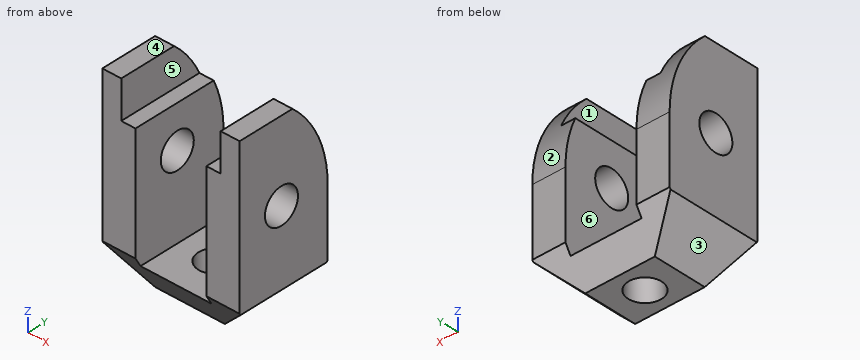
```python
from build123d import *

# Parameters (mm, degrees)
SKETCH1_R                           = 7.5
BOSS_EXTRUDE1_DEPTH                 = 58
CUT_EXTRUDE1_DEPTH                  = 107.60206377
CUT_EXTRUDE1_DEPTH_BACK             = 10
SKETCH3_W                           = 30
SKETCH3_H                           = 53
CUT_EXTRUDE3_DEPTH                  = 107.60206377
CUT_EXTRUDE3_DIRECTION_2_REACH      = 108.602
CUT_EXTRUDE3_DIRECTION_2_END_RADIUS = 50
CUT_EXTRUDE4_DEPTH                  = 107.60206377
SKETCH8_R                           = 7
CUT_EXTRUDE5_DEPTH                  = 107.60206377


with BuildPart() as part:
    # Sketch1 → Boss-Extrude1 (new body)
    with BuildSketch(Plane(origin=(0, 0, 0), x_dir=(0, 0, -1), z_dir=(1, 0, 0))):
        with BuildLine():
            Line((0, 0), (65, 0))
            Line((65, 0), (80, 8.660254038))
            Line((80, 8.660254038), (80, 31.339745962))
            Line((80, 31.339745962), (65, 40))
            Line((65, 40), (36.66060556, 40))
            ThreePointArc((36.66060556, 40), (16.66060556, 35.82575695), (0, 24))
            Line((0, 24), (0, 0))
        make_face()
        with Locations(Location((34, 19, 0), (0, 0, 180))):
            Circle(SKETCH1_R, mode=Mode.SUBTRACT)
    extrude(amount=BOSS_EXTRUDE1_DEPTH)

    # Sketch3 → Cut-Extrude1 (cut, two sides: drawn at the far end of the back side and taken through both)
    with BuildSketch(Plane(origin=(0, 0, 0), x_dir=(1, 0, 0), z_dir=(0, 1, 0)).offset(-CUT_EXTRUDE1_DEPTH_BACK)):
        with Locations((29, 42.5)):
            Rectangle(SKETCH3_W, SKETCH3_H)
    extrude(amount=CUT_EXTRUDE1_DEPTH + CUT_EXTRUDE1_DEPTH_BACK, mode=Mode.SUBTRACT)

    # Sketch5 → Cut-Extrude3 (cut)
    with BuildSketch(Plane(origin=(0, 0, 0), x_dir=(1, 0, 0), z_dir=(0, 1, 0))):
        Polygon((29, 0), (29, 16), (14, 16), (8, 16), (8, 0), align=None)
        Polygon((44, 16), (29, 16), (29, 0), (50, 0), (50, 16), align=None)
    extrude(amount=-CUT_EXTRUDE3_DEPTH, mode=Mode.SUBTRACT)

    # Cut-Extrude3 direction 2: up to this cylinder (the profile starts inside it)
    cut_extrude3_direction_2_end = Plane(origin=(29, -10, -36.66060556), z_dir=(-1, 0, 0)) * Cylinder(CUT_EXTRUDE3_DIRECTION_2_END_RADIUS, 339.204, mode=Mode.PRIVATE)
    # Sketch5 → Cut-Extrude3 direction 2 (cut, up to the surface)
    with BuildSketch(Plane(origin=(0, 0, 0), x_dir=(1, 0, 0), z_dir=(0, 1, 0)), mode=Mode.PRIVATE) as cut_extrude3_direction_2_sk1:
        Polygon((29, 0), (29, 16), (14, 16), (8, 16), (8, 0), align=None)
    cut_extrude3_direction_2_tool1 = extrude(cut_extrude3_direction_2_sk1.sketch, amount=CUT_EXTRUDE3_DIRECTION_2_REACH, mode=Mode.PRIVATE) & cut_extrude3_direction_2_end
    add(cut_extrude3_direction_2_tool1.solids().sort_by_distance((18.5, 0, -8))[0], mode=Mode.SUBTRACT)
    # Sketch5 → Cut-Extrude3 direction 2 (cut, up to the surface)
    with BuildSketch(Plane(origin=(0, 0, 0), x_dir=(1, 0, 0), z_dir=(0, 1, 0)), mode=Mode.PRIVATE) as cut_extrude3_direction_2_sk2:
        Polygon((44, 16), (29, 16), (29, 0), (50, 0), (50, 16), align=None)
    cut_extrude3_direction_2_tool2 = extrude(cut_extrude3_direction_2_sk2.sketch, amount=CUT_EXTRUDE3_DIRECTION_2_REACH, mode=Mode.PRIVATE) & cut_extrude3_direction_2_end
    add(cut_extrude3_direction_2_tool2.solids().sort_by_distance((39.5, 0, -8))[0], mode=Mode.SUBTRACT)

    # Sketch7 → Cut-Extrude4 (cut, through all)
    with BuildSketch(Plane(origin=(0, 0, 0), x_dir=(1, 0, 0), z_dir=(0, 1, 0))):
        Polygon((0, 65.69666313), (14.30333687, 80), (0, 80), align=None)
        Polygon((58, 65.69666313), (43.69666313, 80), (58, 80), align=None)
    extrude(amount=CUT_EXTRUDE4_DEPTH, mode=Mode.SUBTRACT)

    # Sketch8 → Cut-Extrude5 (cut, through all)
    with BuildSketch(Plane(origin=(0, 0, -80), x_dir=(-1, 0, 0), z_dir=(0, 0, -1))):
        with Locations((-29, 20)):
            Circle(SKETCH8_R)
    extrude(amount=-CUT_EXTRUDE5_DEPTH, mode=Mode.SUBTRACT)


solid = part.part
```
The model under review builds one solid part; all positions refer to its coordinate system, in mm. Face numbers are marked on the shaded views. A direction names the side the tool comes from. Give positions to 0.01 mm unless a question says otherwise; leave off trailing zeros. Loops run counter-clockwise (first coordinate to the right, second up) from the corner with the lowest first, then second, coordinate; pieces in that order, holes last. Notation, with made-up numbers: (50.25, -13.75) - (76.25, -13.75) arc R26 ccw to (76.25, 24.25) - close; hole circle Ø9 at (23, 0.5). An arc over 180 degrees is marked (long way). Answer as a JSON object with one key per item and string values.
Q1. Add section D-D on x = 10. State the section outline as (y, z) points, plus the area to 3 significant figures.
Worked out:
{"outline": "(0, -65) - (6.18, -75.7) - (33.82, -75.7) - (40, -65) - (40, -36.66) arc R50 ccw to (35.53, -16) - (0, -16) - close; hole circle Ø15 at (19, -34)", "area": "2,110 mm^2"}
Q2. For the marked faces 1 and 2, list the 3-axis set-ups (+Z, -Z, +X, -X, +Y, -Y) from which the entire face can be reached by the end or side of a thin tool; tool diameter is ignored.
Worked out:
{"face 1": "+Z, +Y, -Y", "face 2": "+Z, +X, -X, +Y"}
Q3. Insertion check: pin 1 (17 mm diameter, centred on y = 19, z = -34, fed in from -X); pin 2 (12 mm diameter, centred on y = 19, z = -34, fed in from +X); pin 3 (1.8 mm diameter, centred on x = 10.5, y = 26, fed in from +Z). Each pin has a flat end and moves straight along its axis. Give the tip position at first contact, or say it passes through.
Worked out:
{"pin 1": "stops at x = 0", "pin 2": "passes through", "pin 3": "stops at z = -16"}
Q4. To check wall thickness, follow line 1 along X through (y, z) = (26, -11.5); line 2 along X through (y, z) = (29.5, -33); line 3 along Y through (x, z) = (12, -37). State the ranges of each line that lie inside material, in increasing order.
Worked out:
{"line 1": "x = 0 to 8, 50 to 58", "line 2": "x = 0 to 14, 44 to 58", "line 3": "y = 0 to 12.13, 25.87 to 40"}
Q5. Add section A-A on x = 29. State the section outline as (y, z) points, plus the area to 3 significant figures.
Worked out:
{"outline": "(2.31, -69) - (8.66, -80) - (13, -80) - (13, -69) - close; (27, -80) - (31.34, -80) - (37.69, -69) - (27, -69) - close", "area": "165 mm^2"}
Q6. Mouldability with a two-part tool opening along X and no side actions: class the marked faces 3, 4, 5 and 6 as +X half, -X half, draft (parallel to the pull), parting line (faces both ways), or undercut.
Worked out:
{"face 3": "-X half", "face 4": "draft", "face 5": "undercut", "face 6": "undercut"}
Q7. Add section C-C on y = 18. State the section outline as (x, z) points, plus the area to 3 significant figures.
Worked out:
{"outline": "(0, -65.7) - (14.3, -80) - (22.29, -80) - (22.29, -69) - (14, -69) - (14, -41.43) - (0, -41.43) - close; (0, -26.57) - (14, -26.57) - (14, -16) - (8, -16) - (8, 0) - (0, 0) - close; (35.71, -80) - (43.7, -80) - (58, -65.7) - (58, -41.43) - (44, -41.43) - (44, -69) - (35.71, -69) - close; (44, -26.57) - (58, -26.57) - (58, 0) - (50, 0) - (50, -16) - (44, -16) - close", "area": "1,610 mm^2"}
Q8. Add section B-B on z = -19. State the section outline as (x, y) points.
Worked out:
{"outline": "(0, 0) - (14, 0) - (14, 36.78) - (0, 36.78) - close; (44, 0) - (58, 0) - (58, 36.78) - (44, 36.78) - close"}
